```python
from build123d import *

# Parameters (mm, degrees)
SKETCH1_R           = 7.5
BOSS_EXTRUDE1_DEPTH = 3
CHAMFER3_SIZE       = 0.2
CHAMFER3_SIZE2      = 0.549495484


with BuildPart() as part:
    # Sketch1 → Boss-Extrude1 (new body)
    with BuildSketch(Plane.XY):
        Circle(SKETCH1_R)
        with BuildLine():
            Line((-2.7, -1.809005252), (-2.7, 1.809005252))
            ThreePointArc((-2.7, 1.809005252), (3.25, 0), (-2.7, -1.809005252))
        make_face(mode=Mode.SUBTRACT)
    extrude(amount=BOSS_EXTRUDE1_DEPTH)

    # Chamfer3
    chamfer3_edges = [part.edges().sort_by_distance(p)[0] for p in [
        (3.25, 0, 3),
        (-2.7, 0, 3),
    ]]
    chamfer3_side = [part.faces().sort_by_distance(p)[0] for p in [
        (-7.287867966, 0, 3),
    ]]
    chamfer(chamfer3_edges, length=CHAMFER3_SIZE, length2=CHAMFER3_SIZE2, reference=chamfer3_side[0])


solid = part.part
```
Build history of the part. All positions in model axes, mm. A direction names the side the tool comes from. Coordinates: 2 decimals unless noted, no trailing zeros. Write each loop counter-clockwise with the first axis right and the second up, starting at its lowest first coordinate (ties: lowest second). Pieces come first, ordered by that corner, then holes.
1. Band-saw the part on A-A, the plane y = 0. Give the cut face in (x, z).
Answer block:
outline: (-7.5, 0) - (-2.7, 0) - (-2.7, 2.45) - (-2.9, 3) - (-7.5, 3) - close; (3.25, 0) - (7.5, 0) - (7.5, 3) - (3.45, 3) - (3.25, 2.45) - close
2. Drop flat-ended pins along their axis: pin 1 (1 mm diameter, centred on y = 1, z = 1.5, fed in from -X); pin 2 (1.5 mm diameter, centred on y = -4.5, z = 2, fed in from -X); pin 3 (0.7 mm diameter, centred on y = -0.5, z = 1.5, fed in from +X). Give the stop position or say it passes through.
Answer block:
pin 1: stops at x = -7.48
pin 2: stops at x = -6.5
pin 3: stops at x = 7.5
3. Band-saw the part on D-D, the plane y = -4.5. Give the cut face in (x, z), and give its area (3 significant figures).
Answer block:
outline: (-6, 0) - (6, 0) - (6, 3) - (-6, 3) - close
area: 36.0 mm2
4. Pull direction X, two halves, no side cores. Call faces 3 (the cylindrical face through (-7.493, 0.33, 1.479)), 4 (the flat face through (2, -3, 0)), 5 (the conical face through (3.302, 0.119, 2.599)): released by +X, released by -X, zero draft, split by the parting line, or undercut.
Answer block:
face 3: split by the parting line
face 4: zero draft
face 5: undercut
5. Band-saw the part on B-B, the plane x = 0. Give the cut face in (y, z).
Answer block:
outline: (-7.5, 0) - (-3.25, 0) - (-3.25, 2.45) - (-3.45, 3) - (-7.5, 3) - close; (3.25, 0) - (7.5, 0) - (7.5, 3) - (3.45, 3) - (3.25, 2.45) - close
6. Drill centre lines: probe 1 along Y at (x, z) = (0, 1.25); probe 2 along Y at (x, z) = (6.75, 2.55); probe 3 along Y at (x, z) = (5.5, 1.8). Where is each one in solid material? Low to high.
Answer block:
probe 1: y = -7.5 to -3.25, 3.25 to 7.5
probe 2: y = -3.27 to 3.27
probe 3: y = -5.1 to 5.1
7. Band-saw the part on C-C, the plane z = 1.8. Give the cut face in (x, y), and give its area (3 significant figures).
Answer block:
outline: circle Ø15 at (0, 0); hole (-2.7, -1.81) arc R3.25 ccw (long way) to (-2.7, 1.81) - close
area: 145 mm2
8. 3-axis set-ups, long thin cutter, end or side, ignore diameter. For faces 1 (the flat face through (2, -3, 3)), 2 (the flat face through (-2.7, 0, 1)): which of +Z, -Z, +X, -X, +Y, -Y reach the whole face in a straight line?
Answer block:
face 1: +Z, +X, -X, +Y, -Y
face 2: +Z, -Z
